from build123d import *

# Parameters (mm, degrees)
SKETCH1_W           = 61.169
SKETCH1_H           = 44.752
BOSS_EXTRUDE1_DEPTH = 4
SKETCH2_W           = 34
SKETCH2_H           = 34
BOSS_EXTRUDE2_DEPTH = 6
CUT_EXTRUDE1_DEPTH  = 4
SKETCH4_R           = 3.969265512
CUT_EXTRUDE2_DEPTH  = 77.028863368
FILLET1_R           = 18
FILLET2_R           = 18
FILLET3_R           = 18
FILLET4_START       = 4
FILLET4_DEPTH       = 6
SKETCH5_R           = 1.25
CUT_EXTRUDE3_DEPTH  = 77.028863368
FILLET5_R           = 2
FILLET6_R           = 2
FILLET7_R           = 2
FILLET8_R           = 2


with BuildPart() as part:
    # Sketch1 → Boss-Extrude1 (new body)
    with BuildSketch(Plane.XY):
        with Locations((30.5845, 22.376)):
            Rectangle(SKETCH1_W, SKETCH1_H)
    extrude(amount=BOSS_EXTRUDE1_DEPTH)

    # Sketch2 → Boss-Extrude2 (add)
    with BuildSketch(Plane.XY.offset(4)):
        with Locations((30.5845, 22.376)):
            Rectangle(SKETCH2_W, SKETCH2_H)
    extrude(amount=BOSS_EXTRUDE2_DEPTH)

    # Sketch3 → Cut-Extrude1 (cut)
    with BuildSketch(Plane.XY.offset(10)):
        with BuildLine():
            Line((27.356049636, 38.095217862), (27.01861523, 26.313045343))
            ThreePointArc((27.01861523, 26.313045343), (25.684503943, 23.381545743), (27.010272743, 20.446263829))
            Line((27.010272743, 20.446263829), (27.309152271, 8.890153737))
            ThreePointArc((27.309152271, 8.890153737), (29.453459694, 6.929735982), (31.806869101, 8.633483691))
            Line((31.806869101, 8.633483691), (32.149278144, 20.437988245))
            ThreePointArc((32.149278144, 20.437988245), (33.484497114, 23.371255165), (32.156419459, 26.307762319))
            Line((32.156419459, 26.307762319), (31.846569585, 37.941982205))
            ThreePointArc((31.846569585, 37.941982205), (29.662940134, 39.824662034), (27.356049636, 38.095217862))
        make_face()
    extrude(amount=-CUT_EXTRUDE1_DEPTH, mode=Mode.SUBTRACT)

    # Sketch4 → Cut-Extrude2 (cut, through all)
    with BuildSketch(Plane.XY.offset(6)):
        with Locations((28.564891977, 22.86990875)):
            Circle(SKETCH4_R)
    extrude(amount=-CUT_EXTRUDE2_DEPTH, mode=Mode.SUBTRACT)

    # Fillet1
    # the kernel refuses this fillet: 18 mm, written as the material it takes off along each edge
    with BuildSketch(Plane(origin=(13.5845, 39.376, 4), x_dir=(0, -1, 0), z_dir=(0, 0, 1))) as fillet1_piece_1:
        with BuildLine():
            CenterArc((FILLET1_R, FILLET1_R), FILLET1_R, 180, 90)
            Line((0, FILLET1_R), (0, 0))
            Line((0, 0), (FILLET1_R, 0))
        make_face()
    extrude(amount=51, mode=Mode.SUBTRACT)

    # Fillet2
    # the kernel refuses this fillet: 18 mm, written as the material it takes off along each edge
    with BuildSketch(Plane(origin=(47.5845, 39.376, 4), x_dir=(0, -1, 0), z_dir=(0, 0, 1))) as fillet2_piece_1:
        with BuildLine():
            CenterArc((17.88854382, -18), FILLET2_R, 90, 83.620629792)
            Line((0, -16), (0, 0))
            Line((0, 0), (17.88854382, 0))
        make_face()
    extrude(amount=50.72135955, mode=Mode.SUBTRACT)

    # Fillet3
    # the kernel refuses this fillet: 18 mm, written as the material it takes off along each edge
    with BuildSketch(Plane(origin=(13.5845, 5.376, 4), x_dir=(0, 1, 0), z_dir=(0, 0, 1))) as fillet3_piece_1:
        with BuildLine():
            CenterArc((18, -17.88854382), FILLET3_R, 96.379370208, 83.620629792)
            Line((0, -17.88854382), (0, 0))
            Line((0, 0), (16, 0))
        make_face()
    extrude(amount=50.72135955, mode=Mode.SUBTRACT)

    # Fillet4: read off the stored shape, not the designer's step
    # Fillet4 outline → Fillet4 (cut)
    with BuildSketch(Plane.XY.offset(FILLET4_START)):
        with BuildLine():
            ThreePointArc((47.5845, 21.48745618), (42.054418725, 10.300490896), (30.578445069, 5.398244493))
            ThreePointArc((30.578445069, 5.398244493), (31.025606187, 5.381561983), (31.47304382, 5.376))
            Line((31.47304382, 5.376), (47.5845, 5.376))
            Line((47.5845, 5.376), (47.5845, 21.48745618))
        make_face()
    extrude(amount=FILLET4_DEPTH, mode=Mode.SUBTRACT)

    # Sketch5 → Cut-Extrude3 (cut, through all)
    with BuildSketch(Plane.XY.offset(4)):
        with Locations((4, 40.752)):
            Circle(SKETCH5_R)
        with Locations((57.169, 40.752)):
            Circle(SKETCH5_R)
        with Locations((4, 4)):
            Circle(SKETCH5_R)
        with Locations((57.169, 4)):
            Circle(SKETCH5_R)
    extrude(amount=-CUT_EXTRUDE3_DEPTH, mode=Mode.SUBTRACT)

    # Fillet5
    fillet5_edges = [part.edges().sort_by_distance(p)[0] for p in [
        (30.5845, 0, 4),
    ]]
    fillet(fillet5_edges, radius=FILLET5_R)

    # Fillet6
    fillet6_edges = [part.edges().sort_by_distance(p)[0] for p in [
        (61.169, 23.376, 4),
        (61.169, 0, 1),
        (61.169, 0.585786438, 3.414213562),
    ]]
    fillet(fillet6_edges, radius=FILLET6_R)

    # Fillet7
    fillet7_edges = [part.edges().sort_by_distance(p)[0] for p in [
        (0, 23.376, 4),
        (0, 0, 1),
        (0, 0.585786438, 3.414213562),
    ]]
    fillet(fillet7_edges, radius=FILLET7_R)

    # Fillet8
    fillet8_edges = [part.edges().sort_by_distance(p)[0] for p in [
        (61.169, 44.752, 1),
        (60.583213562, 44.752, 3.414213562),
        (0, 44.752, 1),
        (30.5845, 44.752, 4),
        (0.585786438, 44.752, 3.414213562),
    ]]
    fillet(fillet8_edges, radius=FILLET8_R)


solid = part.part
CAD build for the part. Positions are in the model's coordinates, mm. A direction names the side the tool comes from. Round coordinates to 2 decimals unless told otherwise and drop trailing zeros. Loops run counter-clockwise (first coordinate to the right, second up) from the corner with the lowest first, then second, coordinate; pieces in that order, holes last.
(1) Cut at B-B (x = 4). Give the cut face in (y, z), plus the area to 3 significant figures.
(2) Two-plate mould, pull along X, no slides. Class faces 1 (the cylindrical face through (0.57, 0.6, 1.01)), 2 (the flat face through (30, 28, 0)), 3 (the flat face through (33, 23, 6)): +X half, -X half, draft (parallel to the pull), parting line (faces both ways), or undercut.
(3) Which spindle directions (+Z, -Z, +X, -X, +Y, -Y) get a long thin tool onto all of the face, cutting with end or side? Do faces 4 (the cylindrical face through (18.997, 34.243, 6.958)), 5 (the flat face through (43, 36, 4)), 6 (the flat face through (25.5, 22.1, 6)), 7 (the cylindrical face through (25.685, 23.428, 8.028)), 8 (the cylindrical face through (19, 10.4, 7)). Say none if no direction does.
(4) Drop flat-ended pins along their axis: pin 1 (6 mm diameter, centred on y = 39.5, z = 6, fed in from +X); pin 2 (4 mm diameter, centred on x = 4, y = 4, fed in from +Z). Give the stop position or say it passes through.
(5) Wall check: line 1 along X through (y, z) = (23, 1.25); line 2 along Z through (x, y) = (49.5, 13.5); line 3 along X through (y, z) = (5, 2.75). Give the ranges that are in metal, low to high.
(6) Cut at D-D (y = 28.5). Give the cut face in (x, z).
(7) Cut at C-C (x = 19). Give the cut face in (y, z), plus the area to 3 significant figures.
(8) Cut at A-A (y = 4). Give the cut face in (x, z), plus the area to 3 significant figures.
Findings below:
1. outline: (0, 0) - (2.75, 0) - (2.75, 4) - (2, 4) arc R2 ccw to (0, 2) - close; (5.25, 0) - (39.5, 0) - (39.5, 4) - (5.25, 4) - close; (42, 0) - (44.75, 0) - (44.75, 2) arc R2 ccw to (42.75, 4) - (42, 4) - close
1. area: 157 mm2
2. face 1: -X half
2. face 2: draft
2. face 3: undercut
3. face 4: +Z, -X, +Y
3. face 5: +Z
3. face 6: -Z
3. face 7: +Z, -Z
3. face 8: +Z, -X, -Y
4. pin 1: stops at x = 60.9
4. pin 2: stops at z = 4
5. line 1: x = 0 to 24.6, 32.53 to 61.17
5. line 2: z = 0 to 4
5. line 3: x = 0.15 to 3.25, 4.75 to 56.42, 57.92 to 61.02
6. outline: (0, 0) - (61.17, 0) - (61.17, 2) arc R2 ccw to (59.17, 4) - (46.16, 4) - (46.16, 10) - (32.1, 10) - (32.1, 6) - (27.08, 6) - (27.08, 10) - (15.05, 10) - (15.05, 4) - (2, 4) arc R2 ccw to (0, 2) - close
7. outline: (0, 0) - (44.75, 0) - (44.75, 2) arc R2 ccw to (42.75, 4) - (34.25, 4) - (34.25, 10) - (10.4, 10) - (10.4, 4) - (2, 4) arc R2 ccw to (0, 2) - close
7. area: 320 mm2
8. outline: (0, 0) - (2.75, 0) - (2.75, 4) - (2, 4) arc R2 ccw to (0, 2) - close; (5.25, 0) - (55.92, 0) - (55.92, 4) - (5.25, 4) - close; (58.42, 0) - (61.17, 0) - (61.17, 2) arc R2 ccw to (59.17, 4) - (58.42, 4) - close
8. area: 223 mm2
